Could you check a few things on this drawing? It's one solid part, dimensions in mm from its lowest x, y, z. Coordinates: 2 decimals unless noted, no trailing zeros. Loops run counter-clockwise (first coordinate to the right, second up) from the corner with the lowest first, then second, coordinate; pieces in that order, holes last. Notation, with made-up numbers: (66, 14) -> (124, 14) arc R14 ccw to (124, 21) -> close; hole circle Ø9 at (38, 74.5). An arc over 180 degrees is marked (long way). One line per question, with ' | ' between items.
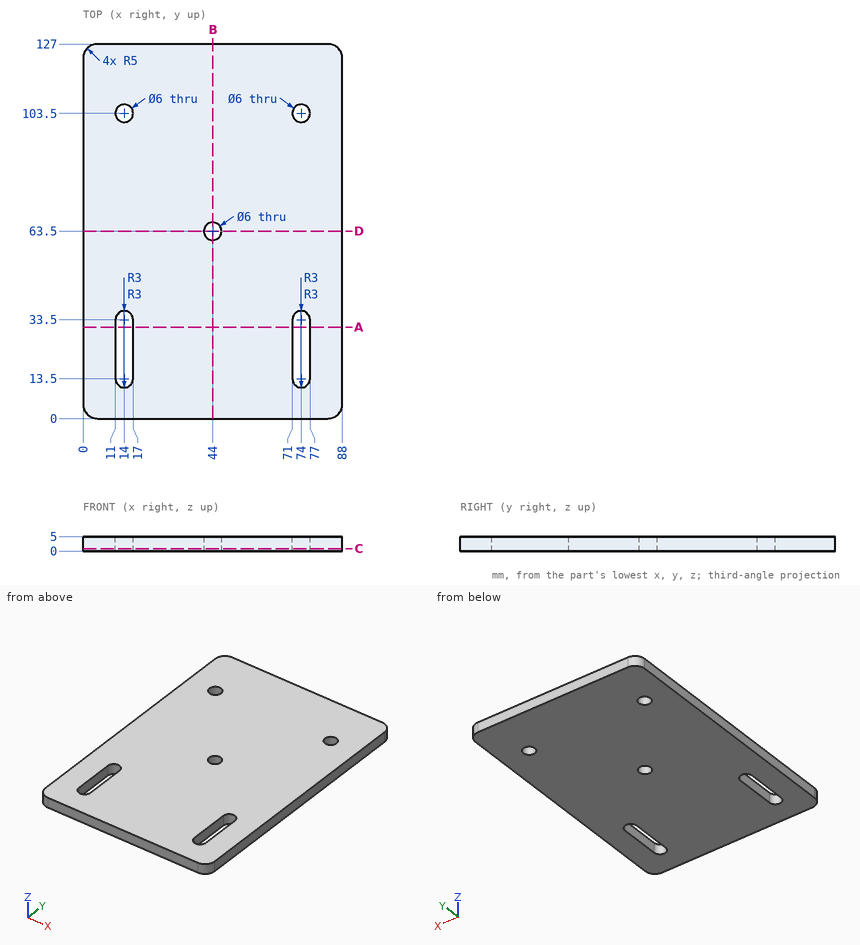
1) I'm going to push a flat-ended pin straight in: pin 1 Ø5 at (x, y) = (44, 63.5) entering from -Z. Where does the tip first touch, or does it pass through?
Data:
pin 1: through
2) If we section it at D-D on y = 63.5: Please give me the cut outline in (x, z), and give its area (3 significant figures).
Data:
outline: (0, 0) -> (41, 0) -> (41, 5) -> (0, 5) -> close; (47, 0) -> (88, 0) -> (88, 5) -> (47, 5) -> close | area: 410 mm²
3) If we section it at B-B on x = 44: Please give me the cut outline in (y, z), and give its area (3 significant figures).
Data:
outline: (0, 0) -> (60.5, 0) -> (60.5, 5) -> (0, 5) -> close; (66.5, 0) -> (127, 0) -> (127, 5) -> (66.5, 5) -> close | area: 605 mm²
4) If we section it at A-A on y = 31: Please give me the cut outline in (x, z), and give its area (3 significant figures).
Data:
outline: (0, 0) -> (11, 0) -> (11, 5) -> (0, 5) -> close; (17, 0) -> (71, 0) -> (71, 5) -> (17, 5) -> close; (77, 0) -> (88, 0) -> (88, 5) -> (77, 5) -> close | area: 380 mm²
5) I need wall thicknesses on line 1 along Y through (x, z) = (74, 1); line 2 along X through (y, z) = (20, 3.4); line 3 along Y through (x, z) = (44, 1.35). Which ranges of each line are inside material? Lowest first, please. Write a range as from..to.
Data:
line 1: 0..10.5, 36.5..100.5, 106.5..127 | line 2: 0..11, 17..71, 77..88 | line 3: 0..60.5, 66.5..127
6) If we section it at C-C on z = 0.85: Please give me the cut outline in (x, y), and give its area (3 significant figures).
Data:
outline: (0, 5) arc R5 ccw to (5, 0) -> (83, 0) arc R5 ccw to (88, 5) -> (88, 122) arc R5 ccw to (83, 127) -> (5, 127) arc R5 ccw to (0, 122) -> close; hole (11, 13.5) arc R3 ccw to (17, 13.5) -> (17, 33.5) arc R3 ccw to (11, 33.5) -> close; hole circle Ø6 at (14, 103.5); hole circle Ø6 at (44, 63.5); hole (71, 13.5) arc R3 ccw to (77, 13.5) -> (77, 33.5) arc R3 ccw to (71, 33.5) -> close; hole circle Ø6 at (74, 103.5) | area: 10,800 mm²
